Design review of the part built by this model. Coordinates are the model's own, in mm. A direction names the side the tool comes from. Coordinates: 2 decimals unless noted, no trailing zeros. Order: outer loops, then holes, each group sorted by start corner. A loop starts at its lowest first (then second) coordinate and runs counter-clockwise, first axis right, second up. Notation, with made-up numbers: M -27,-20.75 L 9,-20.75 A20 ccw 9,3.25 Z; hole C 77.25,-24.75 d6. An arc over 180 degrees is marked long. Use CSV: the item, a comma, the result in double quotes.
```python
from build123d import *

# Parameters (mm, degrees)
F0_R     = 7.5
F1_DEPTH = 4
F2_R     = 5
F3_DEPTH = 100
F4_W     = 4
F4_H     = 4
F5_DEPTH = 20
F6_W     = 2
F6_H     = 4
F7_DEPTH = 20


with BuildPart() as f1:
    # F0 (on Top) → F1 (new body)
    with BuildSketch(Plane.XY):
        Circle(F0_R)
    extrude(amount=F1_DEPTH)

    # F2 (on Top) → F3 (join)
    with BuildSketch(Plane.XY):
        Circle(F2_R)
    extrude(amount=F3_DEPTH)

    # F4 (on face) → F5 (join)
    with BuildSketch(Plane.XY.offset(100)):
        Rectangle(F4_W, F4_H)
    extrude(amount=F5_DEPTH)

    # F6 (on face) → F7 (join)
    with BuildSketch(Plane.XY.offset(120)):
        Rectangle(F6_W, F6_H)
    extrude(amount=F7_DEPTH)


solid = f1.part
```
(1) Add section B-B on z = 124. State the section outline as (x, y) points, and give its area (3 significant figures).
The answers:
outline,"M -1,-2 L 1,-2 L 1,2 L -1,2 Z"
area,"8.00 mm2"
(2) Add section C-C on z = 48.5. State the section outline as (x, y) points.
The answers:
outline,"C 0,0 d10"
(3) Clearance check with flat-ended pins moving along their axes: P1, Ø1.2, axis at x = 0.5, z = 115.5, coming from the +Y side; P2, Ø3, axis at y = -0.5, z = 111, coming from the +X side; P3, Ø3, axis at x = 0, z = 123.5, coming from the -Y side; P4, Ø1.5, axis at x = -2, z = 125.5, coming from the +Y side. State where each tip first meets the part, or that it passes through.
The answers:
P1,"stops at y = 2"
P2,"stops at x = 2"
P3,"stops at y = -2"
P4,"passes through"
(4) Add section A-A on y = 0. State the section outline as (x, z) points.
The answers:
outline,"M -7.5,0 L 7.5,0 L 7.5,4 L 5,4 L 5,100 L 2,100 L 2,120 L 1,120 L 1,140 L -1,140 L -1,120 L -2,120 L -2,100 L -5,100 L -5,4 L -7.5,4 Z"
(5) For faces 1 (the face through (2, -5, 4)), 2 (the face through (-2, 0, 110)), 3 (the face through (2, 0, 110)), list the 3-axis set-ups (+Z, -Z, +X, -X, +Y, -Y) from which the entire face can be reached by the end or side of a thin tool; tool diameter is ignored.
The answers:
face 1,"+Z"
face 2,"+Z, -X, +Y, -Y"
face 3,"+Z, +X, +Y, -Y"
(6) Wall thickness on probe 1 along Z at (x, y) = (3.25, -6); probe 2 along X at (y, z) = (0, 19.5); probe 3 along Z at (x, y) = (4, -1.75): over which ranges is each line inside the solid? List them lowest first.
The answers:
probe 1,"z = 0 to 4"
probe 2,"x = -5 to 5"
probe 3,"z = 0 to 100"
